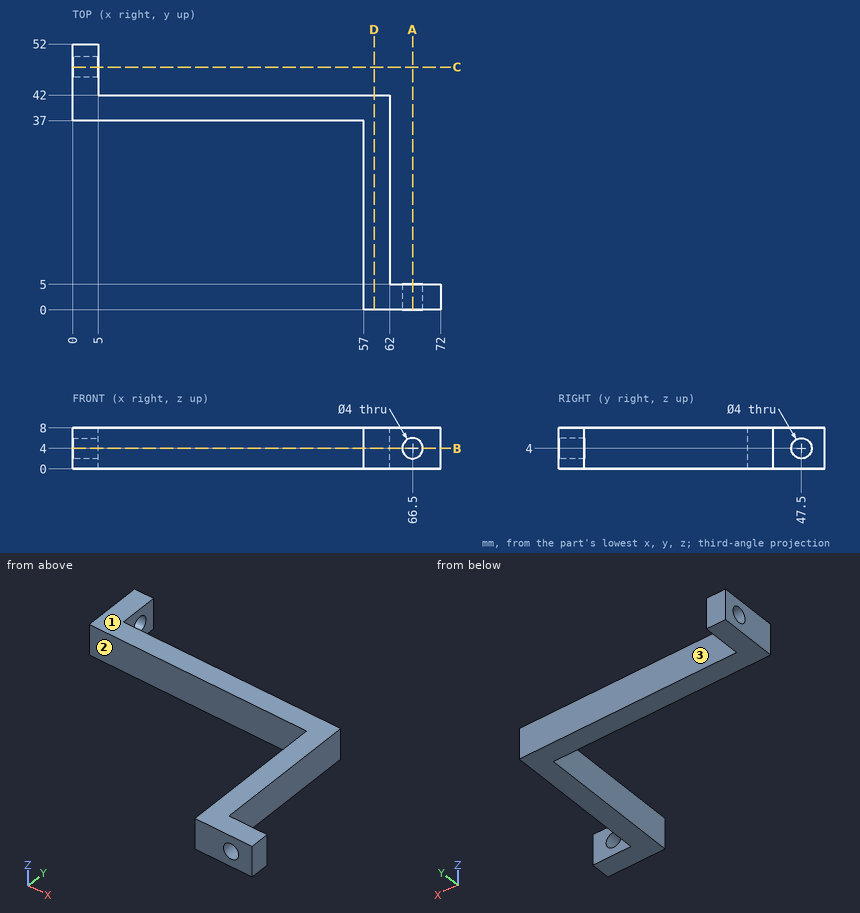
Geometry: see drawing. Coordinates: mm, zero at the bounding-box minimum. A direction names the side the tool comes from. Give positions to 0.01 mm unless a question says otherwise; leave off trailing zeros. Order: outer loops, then holes, each group sorted by start corner. A loop starts at its lowest first (then second) coordinate and runs counter-clockwise, first axis right, second up. Notation, with made-up numbers: (-33, 32.5) - (-8, 32.5) arc R21 ccw to (-8, 60.5) - close; hole circle Ø8 at (20, -36). An arc over 180 degrees is marked (long way). One line per item, written item: value.
1. Cut plane B-B, the plane z = 4. Output: boundary loops of the cut face in (x, y), and give its area (3 significant figures).
Determined:
outline: (0, 37) - (57, 37) - (57, 0) - (64.5, 0) - (64.5, 5) - (62, 5) - (62, 42) - (5, 42) - (5, 45.5) - (0, 45.5) - close; (0, 49.5) - (5, 49.5) - (5, 52) - (0, 52) - close; (68.5, 0) - (72, 0) - (72, 5) - (68.5, 5) - close
area: 555 mm2
2. Pin query (flat end, axial travel): pin 1 Ø2.5 at (y, z) = (47.5, 2) entering from +X; pin 2 Ø1 at (x, z) = (21.5, 5) entering from -Y; pin 3 Ø2.5 at (x, z) = (69, 4.5) entering from +Y; pin 4 Ø3 at (y, z) = (47.5, 4) entering from +X. Return the tip coordinate at first contact, or that it passes through.
Determined:
pin 1: x = 5
pin 2: y = 37
pin 3: y = 5
pin 4: through
3. Reachability of the marked faces 1, 2 and 3 from +Z, -Z, +X, -X, +Y, -Y: full face, straight path, thin tool, end or side. Return the list, or none.
Determined:
face 1: +Z, +X, -X, +Y, -Y
face 2: +Z, -Z, -X, -Y
face 3: +Z, -Z, +X, +Y
4. Line query: probe 1 along Y at (x, z) = (3, 4); probe 2 along X at (y, z) = (35, 7.75); probe 3 along Y at (x, z) = (45, 5). Output: solid intervals per line, ascending.
Determined:
probe 1: 37 to 45.5, 49.5 to 52
probe 2: 57 to 62
probe 3: 37 to 42
5. Cut plane A-A, the plane x = 66.5. Output: boundary loops of the cut face in (y, z).
Determined:
outline: (0, 0) - (5, 0) - (5, 2) - (0, 2) - close; (0, 6) - (5, 6) - (5, 8) - (0, 8) - close
6. Cut plane D-D, the plane x = 59. Output: boundary loops of the cut face in (y, z), and give its area (3 significant figures).
Determined:
outline: (0, 0) - (42, 0) - (42, 8) - (0, 8) - close
area: 336 mm2
